from build123d import *

# Parameters (mm, degrees)
BOSS_EXTRUDE1_DEPTH   = 3.175
CHAMFER1_SIZE         = 1.27
CHAMFER1_SIZE2        = 3.489296323
CHAMFER1_PART_2_SIZE  = 1.27
CHAMFER1_PART_2_SIZE2 = 3.489296323
CHAMFER2_SIZE         = 3.556
CHAMFER2_SIZE2        = 0.952827328


with BuildPart() as part:
    # Sketch1 → Boss-Extrude1 (new body)
    with BuildSketch(Plane(origin=(0, 0, 0), x_dir=(1, 0, 0), z_dir=(0, 1, 0))):
        Polygon((0, 0), (228.6, 0), (213.36, 50.8), (165.1, 50.8), align=None)
    extrude(amount=BOSS_EXTRUDE1_DEPTH)

    # Chamfer1
    chamfer1_edges = [part.edges().sort_by_distance(p)[0] for p in [
        (220.98, 3.175, -25.4),
    ]]
    chamfer1_side = [part.faces().sort_by_distance(p)[0] for p in [
        (220.98, 1.5875, -25.4),
    ]]
    chamfer(chamfer1_edges, length=CHAMFER1_SIZE, length2=CHAMFER1_SIZE2, reference=chamfer1_side[0])

    # Chamfer1 part 2
    chamfer1_part_2_edges = [part.edges().sort_by_distance(p)[0] for p in [
        (82.55, 3.175, -25.4),
    ]]
    chamfer1_part_2_side = [part.faces().sort_by_distance(p)[0] for p in [
        (82.55, 1.5875, -25.4),
    ]]
    chamfer(chamfer1_part_2_edges, length=CHAMFER1_PART_2_SIZE, length2=CHAMFER1_PART_2_SIZE2, reference=chamfer1_part_2_side[0])

    # Chamfer2
    chamfer2_edges = [part.edges().sort_by_distance(p)[0] for p in [
        (220.98, 0, -25.4),
        (82.55, 0, -25.4),
    ]]
    chamfer2_side = [part.faces().sort_by_distance(p)[0] for p in [
        (143.630397554, 0, -19.885015291),
    ]]
    chamfer(chamfer2_edges, length=CHAMFER2_SIZE, length2=CHAMFER2_SIZE2, reference=chamfer2_side[0])


solid = part.part
Design review of the part built by this model. Coordinates are the model's own, in mm. Coordinates: 2 decimals unless noted, no trailing zeros. Write each loop counter-clockwise with the first axis right and the second up, starting at its lowest first coordinate (ties: lowest second). Pieces come first, ordered by that corner, then holes. Notation, with made-up numbers: (-31.75, 61.25) - (-20.75, 61.25) arc R29 ccw to (-20.75, 83.25) - close; hole circle Ø2 at (6.25, 18). An arc over 180 degrees is marked (long way). One line per item, written item: value.
1) To check wall thickness, follow probe 1 along Z at (x, y) = (149, 1.35); probe 2 along Z at (x, y) = (99, 1.9). State the ranges of each line that lie inside material, in increasing order.
Answer sheet:
probe 1: z = -45.85 to 0
probe 2: z = -30.46 to 0
2) Add section C-C (y = 2.5). State the section outline as (x, z) points, plus the area to 3 significant figures.
Answer sheet:
outline: (5.56, 0) - (170.66, -50.8) - (211.65, -50.8) - (226.89, 0) - close
area: 6,660 mm2
3) Add section D-D (x = 94). State the section outline as (y, z) points (3 decimals), plus the area to 3 significant figures.
Answer sheet:
outline: (0, -25.203) - (0.953, -28.923) - (1.905, -28.923) - (3.175, -25.272) - (3.175, 0) - (0, 0) - close
area: 87.7 mm2
4) Mouldability with a two-part tool opening along Y and no side actions: class faces 1 (the face through (221.1, 1.4, -25)), 2 (the face through (219.24, 2.55, -25.03)), 3 (the face through (89.822, 0.483, -25.803)) as +Y half, -Y half, draft (parallel to the pull), parting line (faces both ways), or undercut.
Answer sheet:
face 1: draft
face 2: +Y half
face 3: -Y half
5) Add section B-B (x = 41). State the section outline as (y, z) points (3 decimals).
Answer sheet:
outline: (0, -8.895) - (0.953, -12.615) - (1.905, -12.615) - (3.175, -8.965) - (3.175, 0) - (0, 0) - close
6) Add section A-A (z = -29.5). State the section outline as (x, y) points (3 decimals), plus the area to 3 significant figures.
Answer sheet:
outline: (95.875, 0.953) - (107.967, 0) - (216.037, 0) - (219.75, 0.953) - (219.75, 1.905) - (216.107, 3.175) - (107.74, 3.175) - (95.875, 1.905) - close
area: 376 mm2
7) Insertion check: pin 1 (1.5 mm diameter, centred on x = 143, y = 1.5, fed in from -Z). The pin has a flat end and moves straight along its axis. Give the tip position at first contact, or say it passes through.
Answer sheet:
pin 1: stops at z = -44.23
